from build123d import *

# Parameters (mm, degrees)
CROQUIS1_R              = 1.5
SALIENTE_EXTRUIR1_DEPTH = 1.6
CROQUIS2_W              = 165
CROQUIS2_H              = 100
SALIENTE_EXTRUIR2_DEPTH = 6.8


with BuildPart() as part:
    # Croquis1 → Saliente-Extruir1 (new body)
    with BuildSketch(Plane(origin=(0, 0, 0), x_dir=(1, 0, 0), z_dir=(0, 1, 0))):
        with BuildLine():
            Line((82.5, -58.75), (82.5, 58.75))
            ThreePointArc((82.5, 58.75), (81.621320344, 60.871320344), (79.5, 61.75))
            Line((79.5, 61.75), (77.5, 61.75))
            ThreePointArc((77.5, 61.75), (75.378679656, 60.871320344), (74.5, 58.75))
            Line((74.5, 58.75), (74.5, 53.25))
            Line((74.5, 53.25), (-74.5, 53.25))
            Line((-74.5, 53.25), (-74.5, 58.75))
            ThreePointArc((-74.5, 58.75), (-75.378679656, 60.871320344), (-77.5, 61.75))
            Line((-77.5, 61.75), (-79.5, 61.75))
            ThreePointArc((-79.5, 61.75), (-81.621320344, 60.871320344), (-82.5, 58.75))
            Line((-82.5, 58.75), (-82.5, -58.75))
            ThreePointArc((-82.5, -58.75), (-81.621320344, -60.871320344), (-79.5, -61.75))
            Line((-79.5, -61.75), (-77.5, -61.75))
            ThreePointArc((-77.5, -61.75), (-75.378679656, -60.871320344), (-74.5, -58.75))
            Line((-74.5, -58.75), (-74.5, -53.25))
            Line((-74.5, -53.25), (74.5, -53.25))
            Line((74.5, -53.25), (74.5, -58.75))
            ThreePointArc((74.5, -58.75), (75.378679656, -60.871320344), (77.5, -61.75))
            Line((77.5, -61.75), (79.5, -61.75))
            ThreePointArc((79.5, -61.75), (81.621320344, -60.871320344), (82.5, -58.75))
        make_face()
        with Locations((78.5, 57.5)):
            Circle(CROQUIS1_R, mode=Mode.SUBTRACT)
        with Locations((78.5, -57.5)):
            Circle(CROQUIS1_R, mode=Mode.SUBTRACT)
        with Locations((-78.5, -57.5)):
            Circle(CROQUIS1_R, mode=Mode.SUBTRACT)
        with Locations((-78.5, 57.5)):
            Circle(CROQUIS1_R, mode=Mode.SUBTRACT)
    extrude(amount=SALIENTE_EXTRUIR1_DEPTH)

    # Croquis2 → Saliente-Extruir2 (add)
    with BuildSketch(Plane(origin=(0, 1.6, 0), x_dir=(1, 0, 0), z_dir=(0, 1, 0))):
        with Locations((0, 2.05)):
            Rectangle(CROQUIS2_W, CROQUIS2_H)
    extrude(amount=SALIENTE_EXTRUIR2_DEPTH)


solid = part.part
Build history of the part. All positions in model axes, mm. A direction names the side the tool comes from. Round coordinates to 2 decimals unless told otherwise and drop trailing zeros. Loops run counter-clockwise (first coordinate to the right, second up) from the corner with the lowest first, then second, coordinate; pieces in that order, holes last. Notation, with made-up numbers: (-36.5, -24) -> (8.5, -24) arc R11 ccw to (8.5, -20) -> close; hole circle Ø9 at (16.5, 26.5). An arc over 180 degrees is marked (long way). One line per item, written item: value. Start each with the question number.
Q1. Probe line 1 along X through (y, z) = (1.25, -57.5); line 2 along Z through (x, y) = (-78.5, 0.7); line 3 along Z through (x, y) = (-49.5, 7.5). List the from-to ranges inside material, lowest first.
Q2. Drop flat-ended pins along their axis: pin 1 Ø2 at (x, y) = (-47.5, 1) entering from +Z; pin 2 Ø2 at (x, y) = (27, 6) entering from -Z; pin 3 Ø5 at (x, y) = (40, 6.5) entering from +Z. Give the stop position or say it passes through.
Q3. Cut at C-C on z = 50. List the corners of the cut face in (x, y).
Q4. 3-axis set-ups, long thin cutter, end or side, ignore diameter. For faces 1 (the face through (-1, 1.6, 50)), 2 (the face through (-1, 8.4, -3)), 3 (the face through (-1, 5, -52.05)): which of +Z, -Z, +X, -X, +Y, -Y reach the whole face in a straight line?
Q5. Cut at A-A on x = 21.5. List the corners of the cut face in (y, z).
Q6. Cut at B-B on y = 6.75. List the corners of the cut face in (x, z), plus the area to 3 significant figures.
Computed:
1. line 1: -82.5 to -80, -77 to -74.5, 74.5 to 77, 80 to 82.5
1. line 2: -61.75 to -59, -56 to 56, 59 to 61.75
1. line 3: -52.05 to 47.95
2. pin 1: z = 53.25
2. pin 2: z = -52.05
2. pin 3: z = 47.95
3. outline: (-82.5, 0) -> (82.5, 0) -> (82.5, 1.6) -> (-82.5, 1.6) -> close
4. face 1: +Z, +X, -X, +Y
4. face 2: +Z, -Z, +X, -X, +Y
4. face 3: -Z, +X, -X, +Y
5. outline: (0, -53.25) -> (1.6, -53.25) -> (1.6, -52.05) -> (8.4, -52.05) -> (8.4, 47.95) -> (1.6, 47.95) -> (1.6, 53.25) -> (0, 53.25) -> close
6. outline: (-82.5, -52.05) -> (82.5, -52.05) -> (82.5, 47.95) -> (-82.5, 47.95) -> close
6. area: 16,500 mm²
